Autodesk Inventor part; units mm, degrees
ref_plane "YZ Plane" through (0, 0, 0) normal (1, 0, 0) x (0, 1, 0)
ref_plane "XZ Plane" through (0, 0, 0) normal (0, 1, 0) x (-1, 0, 0)
ref_plane "XY Plane" through (0, 0, 0) normal (0, 0, 1) x (1, 0, 0)
sketch "Sketch1" plane through (0, 0, 0) normal (1, 0, 0) x (0, 1, 0)
  line L0 (0, 0) -> (0, -12.7)
  line L1 (0, 0) -> (41.5212, 59.2984)
  line L2 (41.5212, 59.2984) -> (41.5212, -12.7)
  line L3 (41.5212, -12.7) -> (0, -12.7)
  line L4 (41.5212, 2.0806) -> (41.5212, -12.7)
  line L5 (41.5212, -12.7) -> (66.9212, -12.7)
  line L6 (41.5212, 8.3226) -> (41.5212, -12.7)
  line L7 (41.5212, 0) -> (66.9212, 0)
  line L8 (66.9212, 0) -> (66.9212, -12.7)
  line L9 (66.9212, -12.7) -> (41.5212, -12.7)
  line L10 (41.5212, -12.7) -> (41.5212, 0)
  line L11 (41.5212, -6.35) -> (44.0612, -6.35)
  circle A0 centre (44.0612, -6.35) radius 2.1082
  line L12 (66.9212, -12.7) -> (54.2212, -12.7)
  line L13 (54.2212, -12.7) -> (54.2212, -25.4)
  line L14 (54.2212, -25.4) -> (66.9212, -25.4)
  line L15 (66.9212, -25.4) -> (66.9212, -12.7)
  circle A1 centre (60.5712, -19.05) radius 2.1082
  line L16 (54.2212, 0) -> (66.9212, -12.7)
  line L17 (54.2212, -25.4) -> (41.5212, -12.7)
  line L18 (54.2212, 0) -> (41.5212, 12.7)
  point P0 (41.5212, 8.3226)
  point P1 (41.5212, 0)
  point P2 (41.5212, -12.7)
  dimension "d0" = 12.7
  dimension "d1" = 72.39
  dimension "d3" = 145
  dimension "d20" = 2.54
  dimension "d22" = 4.2164
  dimension "d23" = 12.7
  dimension "d24" = 12.7
  dimension "d25" = 25.4
  dimension "d26" = 25.4
  dimension "d27" = 4.2164
  dimension "d30" = 45
extrude "Extrusion1" add sketch "Sketch1" along normal blind 3.175 contours L1 L2 L3 L0 | L2 L7 L16 L5 | L5 L13 L17 | L18 L7 L2 | L5 L15 L14 L13
fillet "Fillet1" radius 1.5875 1 edges at (1.5875, 41.5212, 59.2984)
fillet "Fillet7" radius 19.05 1 edges at (1.5875, 41.5212, 12.7)
fillet "Fillet8" radius 25.4 1 edges at (1.5875, 41.5212, -12.7)
fillet "Fillet9" radius 3.175 4 edges at (1.5875, 54.2212, -25.4) (1.5875, 66.9212, -25.4) (1.5875, 66.9212, -12.7) (1.5875, 0, -12.7)
fillet "Fillet10" radius 25.4 1 edges at (1.5875, 0, 0)
properties part number "flip out sleds"
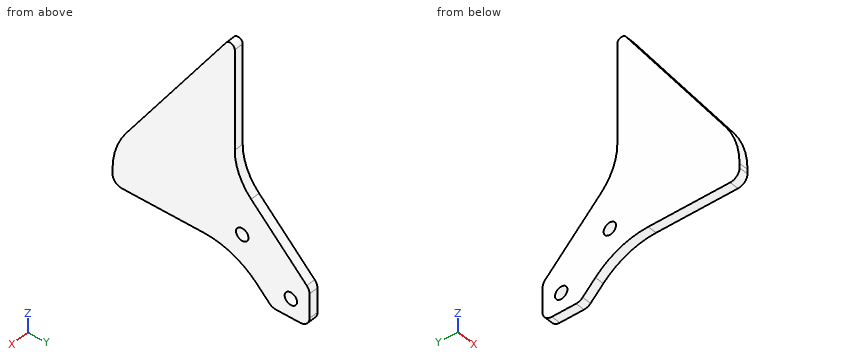
Here's how the part is built. I have some questions about the finished solid (model axes, mm). Coordinates: 2 decimals unless noted, no trailing zeros. Order: outer loops, then holes, each group sorted by start corner. A loop starts at its lowest first (then second) coordinate and runs counter-clockwise, first axis right, second up.
1) Imagine slicing it at C-C on z = -19.05. List the corners of the cut face in (x, y) for me (3 decimals), and give its area (3 significant figures).
2) Imagine slicing it at D-D on z = 13. List the corners of the cut face in (x, y) for me (3 decimals), and give its area (3 significant figures).
3) Imagine slicing it at B-B on z = -6.35. List the corners of the cut face in (x, y) for me (3 decimals), and give its area (3 significant figures).
4) I need wall thicknesses on line 1 (Z direction, x = 2.75, y = 61); line 2 (Y direction, x = 2.15, z = -5); line 3 (Z direction, x = 2.75, y = 29.5). Which ranges of each line are inside material? Lowest first, please.
5) Imagine slicing it at A-A on x = 0.8. State how many separate pieces and enclosed holes the cut face has, and give its area (3 significant figures).
6) Will these pins go through, and if not, where does the flat tip stop? pin 1 (1 mm diameter, centred on x = 1.5, y = 13.5, fed in from -Z); pin 2 (1 mm diameter, centred on x = 2, y = 51.5, fed in from -Z).
Response values:
1. outline: (0, 47.801) - (3.175, 47.801) - (3.175, 58.463) - (0, 58.463) - close; (0, 62.679) - (3.175, 62.679) - (3.175, 66.921) - (0, 66.921) - close
1. area: 47.3 mm2
2. outline: (0, 9.103) - (3.175, 9.103) - (3.175, 43.099) - (0, 43.099) - close
2. area: 108 mm2
3. outline: (0, 0.054) - (3.175, 0.054) - (3.175, 41.953) - (0, 41.953) - close; (0, 46.169) - (3.175, 46.169) - (3.175, 60.571) - (0, 60.571) - close
3. area: 179 mm2
4. line 1: z = -25.4 to -21.11, -16.99 to -6.78
4. line 2: y = 0.18 to 42.44, 45.68 to 59.22
4. line 3: z = -12.7 to 42.13
5. separate pieces: 1
5. enclosed holes: 2
5. area: 2,300 mm2
6. pin 1: stops at z = -12.7
6. pin 2: stops at z = -23.18
